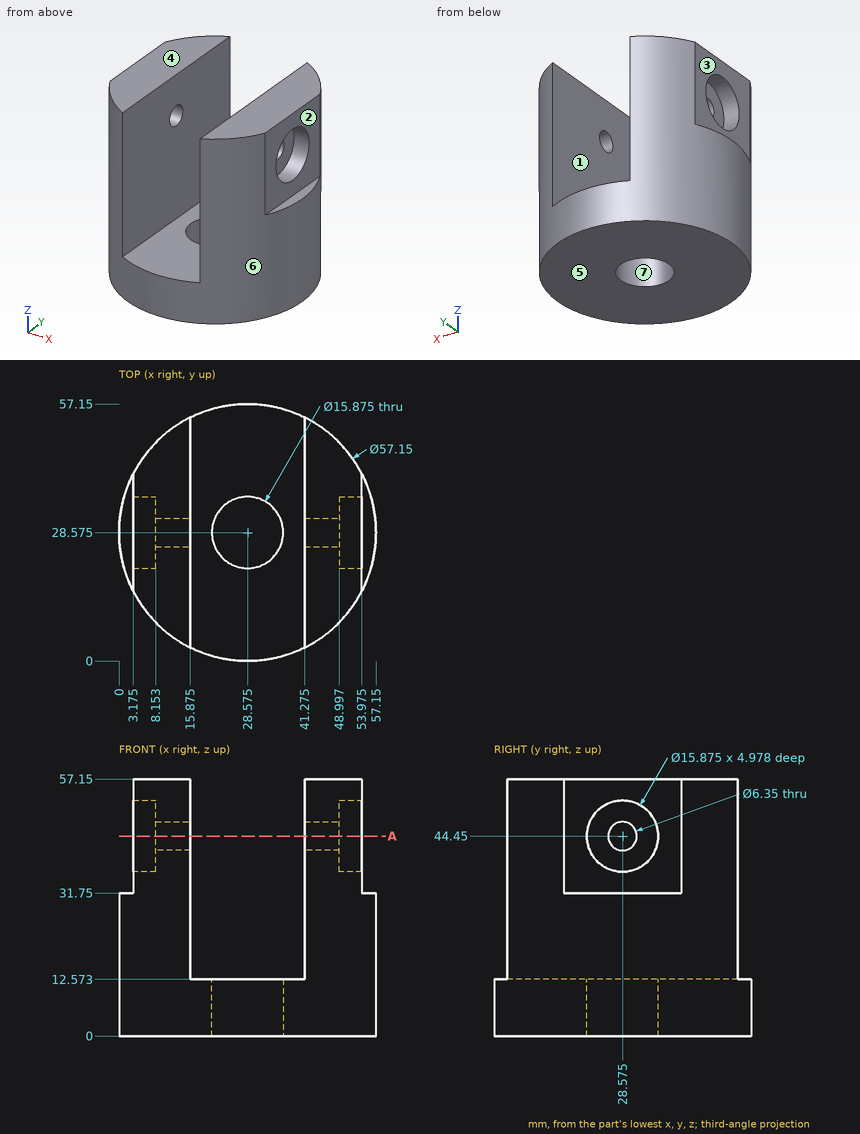
Check sheet for the drawn part. Datum: minimum x, y, z corner. Units: mm. A direction names the side the tool comes from. Give positions to 0.01 mm unless a question says otherwise; leave off trailing zeros. Write item = value, one per line. Start each with the question number.
1) Access from +Z, -Z, +X, -X, +Y, -Y to the whole of each face (thin tool, end or side, straight path). Record for the marked faces 1, 2, 3 and 4.
2) Draft check along Y on the marked faces 5, 6 and 7. Enter one of: released by +Y, released by -Y, zero draft, split by the parting line, or undercut.
3) Gauge pin test, flat ends, axial feed: pin 1 Ø8 at (y, z) = (30.5, 41.5) entering from -X; pin 2 Ø5 at (x, y) = (16.5, 47.5) entering from -Z; pin 3 Ø7.5 at (x, y) = (34.5, 33.5) entering from +Z; pin 4 Ø4 at (y, z) = (12.5, 26) entering from -X. Record the tip position at first contact, or that the pin passes through.
4) Scan lines: L1, parallel to X at y = 30.5, z = 35 (1 decimal); L2, parallel to X at y = 33.5, z = 44.5 (1 decimal); L3, parallel to Z at x = 25.5, y = 47. Record each from-to range of solid material in increasing order.
5) Section check A-A (z = 44.45). Count the separate pieces of the cut face and the enclosed holes in it.
Geometry check:
q1.face_1 = +Z, +Y, -Y
q1.face_2 = +Z, +X, +Y, -Y
q1.face_3 = +Z, -X, +Y, -Y
q1.face_4 = +Z, +X, -X, +Y, -Y
q2.face_5 = zero draft
q2.face_6 = split by the parting line
q2.face_7 = undercut
q3.pin_1 = 8.15
q3.pin_2 = 0
q3.pin_3 = 12.57
q3.pin_4 = 3.71
q4.L1 = 3.2 to 15.9, 41.3 to 54
q4.L2 = 8.2 to 15.9, 41.3 to 49
q4.L3 = 0 to 12.57
q5.separate_pieces = 4
q5.enclosed_holes = 0
